Geometry check sheet. Reference: the model listing, model coordinates, mm. A direction names the side the tool comes from. Coordinates: 2 decimals unless noted, no trailing zeros. Write each loop counter-clockwise with the first axis right and the second up, starting at its lowest first coordinate (ties: lowest second). Pieces come first, ordered by that corner, then holes. Notation, with made-up numbers: (-8.75, 51) -> (31.25, 51) arc R20 cw to (31.25, 73) -> close; hole circle Ø11 at (1, 1.5). An arc over 180 degrees is marked (long way). Put each result on its own line as item: value. Start each with the question number.
from build123d import *

# Parameters (mm, degrees)
BASE_FLANGE1_DEPTH = 1
EDGE_FLANGE1_DEPTH = 27
EDGE_FLANGE2_DEPTH = 27
EDGE_FLANGE3_DEPTH = 20
EDGE_FLANGE4_DEPTH = 20
SKETCH18_R         = 1.4
CUT_EXTRUDE1_DEPTH = 136.048103644
SKETCH19_R         = 1.4
CUT_EXTRUDE2_DEPTH = 75.642159258


# Sheet-metal steps are written as plain solids
with BuildPart() as part:
    # Sketch1 → Base-Flange1 (new body)
    with BuildSketch(Plane.XY):
        with BuildLine():
            Line((-30.928932188, 10.5), (34.928932188, 10.5))
            ThreePointArc((34.928932188, 10.5), (36.84234935, 10.880602337), (38.464466094, 11.964466094))
            Line((38.464466094, 11.964466094), (38.535533906, 12.035533906))
            ThreePointArc((38.535533906, 12.035533906), (40.15765065, 13.119397663), (42.071067812, 13.5))
            Line((42.071067812, 13.5), (60, 13.5))
            Line((60, 13.5), (60, -13.5))
            Line((60, -13.5), (-60, -13.5))
            Line((-60, -13.5), (-60, 13.5))
            Line((-60, 13.5), (-38.071067812, 13.5))
            ThreePointArc((-38.071067812, 13.5), (-36.15765065, 13.119397663), (-34.535533906, 12.035533906))
            Line((-34.535533906, 12.035533906), (-34.464466094, 11.964466094))
            ThreePointArc((-34.464466094, 11.964466094), (-32.84234935, 10.880602337), (-30.928932188, 10.5))
        make_face()
    extrude(amount=-BASE_FLANGE1_DEPTH)

    # Edge-Flange1 section (across the edge) → Edge-Flange1 (add)
    with BuildSketch(Plane(origin=(60.7366, 13.5, -1), x_dir=(-1, 0, 0), z_dir=(0, -1, 0))):
        with BuildLine():
            Line((-1, 0.7366), (-1, 47))
            Line((-1, 47), (0, 47))
            Line((0, 47), (0, 0.7366))
            ThreePointArc((0, 0.7366), (0.215745145, 0.215745145), (0.7366, 0))
            Line((0.7366, 0), (0.7366, -1))
            ThreePointArc((0.7366, -1), (-0.491361636, -0.491361636), (-1, 0.7366))
        make_face()
    extrude(amount=EDGE_FLANGE1_DEPTH)

    # Edge-Flange2 section (across the edge) → Edge-Flange2 (add)
    with BuildSketch(Plane(origin=(-60.7366, -13.5, -1), x_dir=(1, 0, 0), z_dir=(0, 1, 0))):
        with BuildLine():
            Line((-1, 0.7366), (-1, 47))
            Line((-1, 47), (0, 47))
            Line((0, 47), (0, 0.7366))
            ThreePointArc((0, 0.7366), (0.215745145, 0.215745145), (0.7366, 0))
            Line((0.7366, 0), (0.7366, -1))
            ThreePointArc((0.7366, -1), (-0.491361636, -0.491361636), (-1, 0.7366))
        make_face()
    extrude(amount=EDGE_FLANGE2_DEPTH)

    # Edge-Flange3 section (across the edge) → Edge-Flange3 (add)
    with BuildSketch(Plane(origin=(35.7366, -14.2366, -1), x_dir=(0, 1, 0), z_dir=(-1, 0, 0))):
        with BuildLine():
            Line((-1, 0.7366), (-1, 30))
            Line((-1, 30), (0, 30))
            Line((0, 30), (0, 0.7366))
            ThreePointArc((0, 0.7366), (0.215745145, 0.215745145), (0.7366, 0))
            Line((0.7366, 0), (0.7366, -1))
            ThreePointArc((0.7366, -1), (-0.491361636, -0.491361636), (-1, 0.7366))
        make_face()
    extrude(amount=EDGE_FLANGE3_DEPTH)

    # Edge-Flange4 section (across the edge) → Edge-Flange4 (add)
    with BuildSketch(Plane(origin=(15.7366, -15.2366, -31.7366), x_dir=(0, 0, 1), z_dir=(1, 0, 0))):
        with BuildLine():
            Line((-1, 0.7366), (-1, 11))
            Line((-1, 11), (0, 11))
            Line((0, 11), (0, 0.7366))
            ThreePointArc((0, 0.7366), (0.215745145, 0.215745145), (0.7366, 0))
            Line((0.7366, 0), (0.7366, -1))
            ThreePointArc((0.7366, -1), (-0.491361636, -0.491361636), (-1, 0.7366))
        make_face()
    extrude(amount=EDGE_FLANGE4_DEPTH)

    # Sketch18 → Cut-Extrude1 (cut, through all)
    with BuildSketch(Plane.ZY.offset(61.7366)):
        Polygon((-48, 9.5), (-44, 13.5), (-48, 13.5), align=None)
        Polygon((-48, -13.5), (-44, -13.5), (-48, -9.5), align=None)
        with Locations((-42, 7.5)):
            Circle(SKETCH18_R)
        with Locations((-42, 0)):
            Circle(SKETCH18_R)
        with Locations((-42, -7.5)):
            Circle(SKETCH18_R)
    extrude(amount=-CUT_EXTRUDE1_DEPTH, mode=Mode.SUBTRACT)

    # Sketch19 → Cut-Extrude2 (cut, through all)
    with BuildSketch(Plane(origin=(0, 0, -32.7366), x_dir=(-1, 0, 0), z_dir=(0, 0, -1))):
        with BuildLine():
            ThreePointArc((-15.7366, -20.2366), (-17.493959313, -24.479240687), (-21.7366, -26.2366))
            Line((-21.7366, -26.2366), (-15.7366, -26.2366))
            Line((-15.7366, -26.2366), (-15.7366, -20.2366))
        make_face()
        with BuildLine():
            ThreePointArc((-29.7366, -26.2366), (-33.979240687, -24.479240687), (-35.7366, -20.2366))
            Line((-35.7366, -20.2366), (-35.7366, -26.2366))
            Line((-35.7366, -26.2366), (-29.7366, -26.2366))
        make_face()
        with Locations((-30.7366, -22.2366)):
            Circle(SKETCH19_R)
        with Locations((-20.7366, -22.2366)):
            Circle(SKETCH19_R)
    extrude(amount=-CUT_EXTRUDE2_DEPTH, mode=Mode.SUBTRACT)


solid = part.part
Item 1: Access from +Z, -Z, +X, -X, +Y, -Y to the whole of each face (thin tool, end or side, straight path). Record for faces 5 (the flat face through (61, -13.5, -12)), 6 (the flat face through (26, -15.237, -16)), 7 (the flat face through (61, 13.5, -12)).
Item 2: Section check B-B, the plane z = -42. Give the number of separate pieces and of enclosed holes in the cut face, and give its area (3 significant figures).
Item 3: Mould release check, pull along X, two halves, no side actions. Record for faces 1 (the flat face through (-61.2, -11.5, -46)), 2 (the flat face through (60.737, 0, -25)), 3 (the flat face through (1, 0, -1)), 4 (the flat face through (15.737, -15, -19)): released by +X, released by -X, zero draft, split by the parting line, or undercut.
Item 4: Go/stop test with flat-tipped pins: P1, Ø8, axis at x = 29.5, y = -18.5, coming from the -Z side; P2, Ø16, axis at x = 29.5, z = -13.5, coming from the +Y side; P3, Ø10, axis at x = 26, z = -14, coming from the -Y side. Record where each tip stops, or that it passes through.
Item 5: Section check C-C, the plane z = -4. Enter the section's corners in (x, y), and give its area (3 significant figures).
Item 6: Section check D-D, the plane y = -4. Enter the section's corners in (x, z), and give its area (3 significant figures).
Item 7: Section check A-A, the plane y = 7.5. Enter the section's corners in (x, z), and give its area (3 significant figures).
Item 8: Scan lines: line 1 along Y through (x, z) = (61.5, -42); line 2 along X through (y, z) = (-4, -37.5); line 3 along Z through (x, y) = (25, -23). Record each from-to range of solid material in increasing order. Write a range as [from, to].
From the geometry:
1. face 5: +Z, -Z, +X, -Y
1. face 6: +Z, +X, -X, -Y
1. face 7: +Z, -Z, +X, -X, +Y
2. separate pieces: 8
2. enclosed holes: 0
2. area: 37.2 mm²
3. face 1: zero draft
3. face 2: undercut
3. face 3: undercut
3. face 4: released by -X
4. P1: z = -32.74
4. P2: y = -14.24
4. P3: y = -15.24
5. outline: (-61.74, -13.5) -> (-60.74, -13.5) -> (-60.74, 13.5) -> (-61.74, 13.5) -> close; (15.74, -15.24) -> (35.74, -15.24) -> (35.74, -14.24) -> (15.74, -14.24) -> close; (60.74, -13.5) -> (61.74, -13.5) -> (61.74, 13.5) -> (60.74, 13.5) -> close
5. area: 74.0 mm²
6. outline: (-61.74, -48) -> (-60.74, -48) -> (-60.74, -1.74) arc R0.74 cw to (-60, -1) -> (60, -1) arc R0.74 cw to (60.74, -1.74) -> (60.74, -48) -> (61.74, -48) -> (61.74, -1.74) arc R1.74 ccw to (60, 0) -> (-60, 0) arc R1.74 ccw to (-61.74, -1.74) -> close
6. area: 216 mm²
7. outline: (-61.74, -48) -> (-60.74, -48) -> (-60.74, -43.4) -> (-61.74, -43.4) -> close; (-61.74, -40.6) -> (-60.74, -40.6) -> (-60.74, -1.74) arc R0.74 cw to (-60, -1) -> (60, -1) arc R0.74 cw to (60.74, -1.74) -> (60.74, -40.6) -> (61.74, -40.6) -> (61.74, -1.74) arc R1.74 ccw to (60, 0) -> (-60, 0) arc R1.74 ccw to (-61.74, -1.74) -> close; (60.74, -48) -> (61.74, -48) -> (61.74, -43.4) -> (60.74, -43.4) -> close
7. area: 211 mm²
8. line 1: [-13.5, -8.9], [-6.1, -1.4], [1.4, 6.1], [8.9, 13.5]
8. line 2: [-61.74, -60.74], [60.74, 61.74]
8. line 3: [-32.74, -31.74]
